Design review of the part built by this model. Coordinates are the model's own, in mm. A direction names the side the tool comes from. Give positions to 0.01 mm unless a question says otherwise; leave off trailing zeros. Write each loop counter-clockwise with the first axis right and the second up, starting at its lowest first coordinate (ties: lowest second). Pieces come first, ordered by that corner, then holes. Notation, with made-up numbers: (-25.75, 20.25) -> (15.25, 20.25) arc R35 cw to (15.25, 58.25) -> close; hole circle Ø1 at (-37, 24.5). An arc over 180 degrees is marked (long way). Answer as a JSON object with one key per item and string values.
```python
from build123d import *

# Parameters (mm, degrees)
SKETCH1_R           = 15
BOSS_EXTRUDE1_DEPTH = 115
SKETCH2_R           = 40
BOSS_EXTRUDE2_DEPTH = 40
BOSS_EXTRUDE3_START = -40
SKETCH3_R           = 40
BOSS_EXTRUDE3_DEPTH = 40
CHAMFER1_SIZE       = 5
FILLET1_R           = 10


with BuildPart() as part:
    # Sketch1 → Boss-Extrude1 (new, symmetric)
    with BuildSketch(Plane(origin=(0, 0, 0), x_dir=(0, 0, -1), z_dir=(1, 0, 0))):
        Circle(SKETCH1_R)
    extrude(amount=BOSS_EXTRUDE1_DEPTH, both=True)

    # Sketch2 → Boss-Extrude2 (add)
    with BuildSketch(Plane(origin=(115, 0, 0), x_dir=(0, 0, -1), z_dir=(1, 0, 0))):
        Circle(SKETCH2_R)
    extrude(amount=-BOSS_EXTRUDE2_DEPTH)

    # Sketch3 → Boss-Extrude3 (add)
    with BuildSketch(Plane.ZY.offset(115).offset(BOSS_EXTRUDE3_START)):
        with Locations(Location((0, 0, 0), (0, 0, 180))):
            Circle(SKETCH3_R)
    extrude(amount=BOSS_EXTRUDE3_DEPTH)

    # Sketch5 → Revolve1 (revolve)
    with BuildSketch(Plane.XY, mode=Mode.PRIVATE) as revolve1_sk:
        with BuildLine():
            Line((-75, 15), (75, 15))
            ThreePointArc((75, 15), (0, 20), (-75, 15))
        make_face()
    revolve(revolve1_sk.sketch.rotate(Axis((-125.396729405, 0, 0), (1, 0, 0)), 90), axis=Axis((-125.396729405, 0, 0), (1, 0, 0)))

    # Chamfer1
    chamfer1_edges = [part.edges().sort_by_distance(p)[0] for p in [
        (-75, 0, 40),
        (-115, 0, 40),
        (75, 0, 40),
        (115, 0, 40),
    ]]
    chamfer(chamfer1_edges, length=CHAMFER1_SIZE)

    # Fillet1
    fillet1_edges = [part.edges().sort_by_distance(p)[0] for p in [
        (75, 0, -15),
        (-75, 0, -15),
    ]]
    fillet(fillet1_edges, radius=FILLET1_R)


solid = part.part
```
(1) For line 1 along X through (y, z) = (-24, 14); line 2 along X through (y, z) = (3, 22); line 3 along Z through (x, y) = (-41, 10), list the stretches that pass through material, from the lowest coordinate up.
Here are the results:
{"line 1": "x = -115 to -75, 75 to 115", "line 2": "x = -115 to -74.12, 74.12 to 115", "line 3": "z = -15.58 to 15.58"}
(2) Clearance check with flat-ended pins moving along their axes: pin 1 (1.5 mm diameter, centred on x = 19.5, z = 6, fed in from +Y); pin 2 (1.5 mm diameter, centred on x = 80, y = 14.5, fed in from +Z); pin 3 (6 mm diameter, centred on x = 39, y = -10, fed in from +Z). State where each tip first meets the part, or that it passes through.
Here are the results:
{"pin 1": "stops at y = 18.95", "pin 2": "stops at z = 37.56", "pin 3": "stops at z = 17.31"}
(3) The part is to be moulded in two halves that separate along X. For faces 3 (the flat face through (115, 0, 0)), 4 (the conical face through (-114.76, 21.44, 27.97)), 5 (the flat face through (-75, -26, -5)), say which applies: +X half, -X half, draft (parallel to the pull), parting line (faces both ways), or undercut.
Here are the results:
{"face 3": "+X half", "face 4": "-X half", "face 5": "undercut"}
(4) We need section A-A, the plane x = 101. State the section outline as (y, z) points, then the cut area to 3 significant figures.
Here are the results:
{"outline": "circle Ø80 at (0, 0)", "area": "5,030 mm²"}
(5) For faces 1 (the conical face through (75.313, 1.553, 35.279)), 2 (the cylindrical face through (95.21, -39.05, 8.67)), list the 3-axis set-ups (+Z, -Z, +X, -X, +Y, -Y) from which the entire face can be reached by the end or side of a thin tool; tool diameter is ignored.
Here are the results:
{"face 1": "none", "face 2": "+X, -X"}
